Verification items for this drawing (mm, ordinates from the low corner). Coordinates: 2 decimals unless noted, no trailing zeros. Order: outer loops, then holes, each group sorted by start corner. A loop starts at its lowest first (then second) coordinate and runs counter-clockwise, first axis right, second up. Notation, with made-up numbers: (-4.5, -33) - (39.5, -33) arc R12 cw to (39.5, -11) - close; hole circle Ø9 at (64.25, -26). An arc over 180 degrees is marked (long way). Use CSV: the item, a comma, the result in double quotes. Start each with the question number.
1) Sectioned sample at B-B, the plane x = 246.5. Record the cut outline in (y, z).
2) Thickness scan on probe 1 along X at (y, z) = (122, 0.5) (1 decimal); probe 2 along X at (y, z) = (74, 0.75); probe 3 along Y at (x, z) = (203.5, 4.5) (1 decimal). Record the ranges inside material, lowest first. Write a range as [from, to].
3) Sectioned sample at A-A, the plane z = 4.5. Record the cut outline in (x, y).
4) Sectioned sample at C-C, the plane y = 146. Record the cut outline in (x, z) (1 decimal).
5) Depth check by flat-ended pin: P1, Ø12, axis at x = 79.5, y = 93.5, coming from the -Z side; P2, Ø1.5, axis at x = 102.5, z = 7.5, coming from the +Y side. Enter the tip coordinate at first touch or a pass-through.
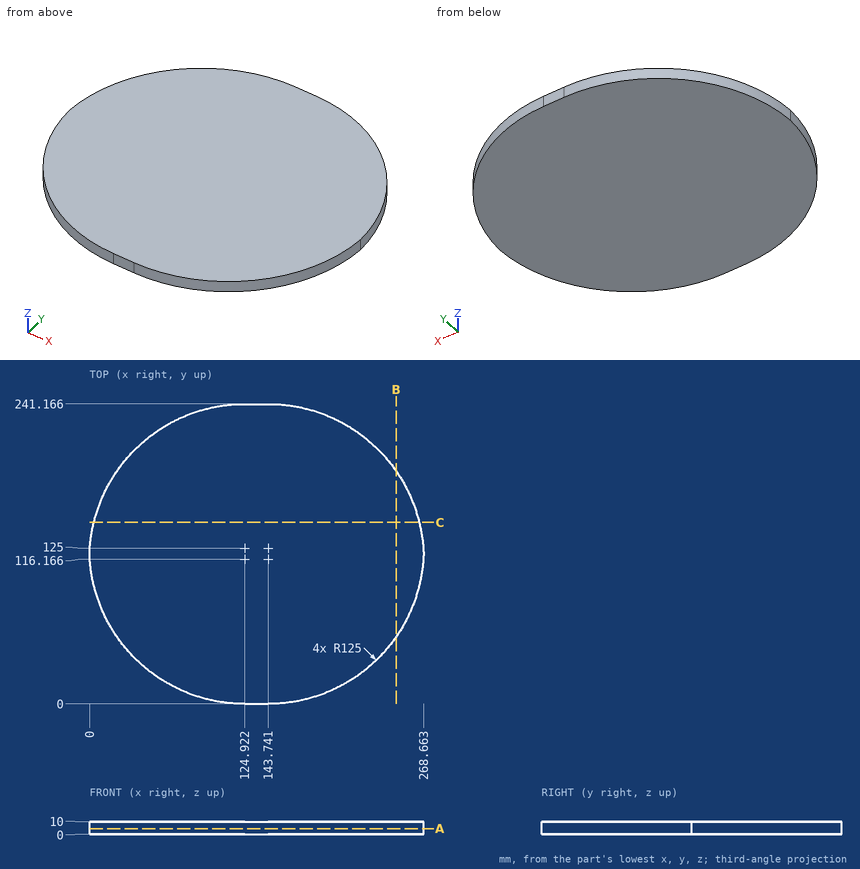
Evaluation:
1,outline,"(53.83, 0) - (187.34, 0) - (187.34, 10) - (53.83, 10) - close"
2,probe 1,"[0.1, 268.6]"
2,probe 2,"[10.8, 257.86]"
2,probe 3,"[15.2, 226]"
3,outline,"(0, 120.58) arc R125 ccw to (124.92, 0) - (143.74, 0) arc R125 ccw to (268.66, 120.58) arc R125 ccw to (143.74, 241.17) - (124.92, 241.17) arc R125 ccw to start"
4,outline,"(3.5, 0) - (265.1, 0) - (265.1, 10) - (3.5, 10) - close"
5,P1,"z = 0"
5,P2,"y = 239.27"
